Input: part model. Units: mm. Frame: model coordinates. Face numbers are marked on the shaded views. A direction names the side the tool comes from. Round coordinates to 2 decimals unless told otherwise and drop trailing zeros. Loops run counter-clockwise (first coordinate to the right, second up) from the corner with the lowest first, then second, coordinate; pieces in that order, holes last. Notation, with made-up numbers: M 18.25,0.25 L 48.25,0.25 A19 ccw 48.25,36.25 Z; hole C -27,24 d6. An arc over 180 degrees is marked long. Put each result on its own line as item: value. Start each with the question number.
1) Section C-C on x = 80. Output: boundary loops of the cut face in (y, z), plus the area to 3 significant figures.
2) Section A-A on y = 0. Output: boundary loops of the cut face in (x, z), plus the area to 3 significant figures.
3) Reachability of the marked faces 1 and 2 from +Z, -Z, +X, -X, +Y, -Y: full face, straight path, thin tool, end or side. Return the list, or none.
4) Line query: probe 1 along X at (y, z) = (7, 26.5); probe 2 along Y at (x, z) = (52.5, -0.5); probe 3 along X at (y, z) = (-1, 31). Output: solid intervals per line, ascending.
5) Draft query along X for the marked faces 3, 4, 5 and 6. Return one class per face: +X half, -X half, draft (parallel to the pull), parting line (faces both ways), or undercut.
6) Section B-B on z = 21.5. Output: boundary loops of the cut face in (x, y), plus the area to 3 significant figures.
7) Pin query (flat end, axial travel): pin 1 (14.5 mm diameter, centred on y = -3, z = 0.5, fed in from -X); pin 2 (1.5 mm diameter, centred on x = 19, z = -4, fed in from -Y); pin 3 (8 mm diameter, centred on x = 7.5, z = 22.5, fed in from +Y). Return the tip coordinate at first contact, or that it passes through.
from build123d import *

# Parameters (mm, degrees)
F1_DEPTH = 36.576
F2_R     = 6.1269141817
F2_R_2   = 5.4449422531
F3_DEPTH = 42.418
F4_DEPTH = 25.4
F5_DEPTH = 25.4
F6_R     = 11.6411765601
F7_DEPTH = 33.528


with BuildPart() as f1:
    # F0 (on Right) → F1 (new body)
    with BuildSketch(Plane.YZ):
        with BuildLine():
            ThreePointArc((-7.3964224414, -6.1888854819), (3.2922075385, -9.0648076628), (9.6441364797, 0))
            ThreePointArc((9.6441364797, 0), (3.2922075385, 9.0648076628), (-7.3964224414, 6.1888854819))
            ThreePointArc((-7.3964224414, 6.1888854819), (-4.251808406, 3.7785340877), (-3.0597214027, 0))
            ThreePointArc((-3.0597214027, 0), (-4.251808406, -3.7785340877), (-7.3964224414, -6.1888854819))
        make_face()
        with BuildLine():
            ThreePointArc((-3.0597214027, 0), (-4.251808406, 3.7785340877), (-7.3964224414, 6.1888854819))
            ThreePointArc((-7.3964224414, 6.1888854819), (-9.6441364797, 0), (-7.3964224414, -6.1888854819))
            ThreePointArc((-7.3964224414, -6.1888854819), (-4.251808406, -3.7785340877), (-3.0597214027, 0))
        make_face()
        with BuildLine():
            ThreePointArc((-7.3964224414, -6.1888854819), (-9.6441364797, 0), (-7.3964224414, 6.1888854819))
            ThreePointArc((-7.3964224414, 6.1888854819), (-16.2285515567, 0), (-7.3964224414, -6.1888854819))
        make_face()
    extrude(amount=F1_DEPTH)

    # F2 (on Top) → F3 (join)
    with BuildSketch(Plane.XY):
        with Locations((10.4273650795, 0)):
            Circle(F2_R)
        with Locations((10.4273650795, 0)):
            Circle(F2_R_2, mode=Mode.SUBTRACT)
    extrude(amount=F3_DEPTH)

    # F4 (add): a face of the model
    f4_faces = [f1.faces().sort_by_distance(p)[0] for p in [
        (36.576, -2.5293914457, 0),
    ]]
    extrude(f4_faces, amount=F4_DEPTH)

    # F5 (add): a face of the model
    f5_faces = [f1.faces().sort_by_distance(p)[0] for p in [
        (61.976, -2.5293914457, 0),
    ]]
    extrude(f5_faces, amount=F5_DEPTH)

    # F6 (on Top) → F7 (join)
    with BuildSketch(Plane.XY):
        with Locations((0, 6.7043649033)):
            Circle(F6_R)
    extrude(amount=F7_DEPTH)


solid = f1.part
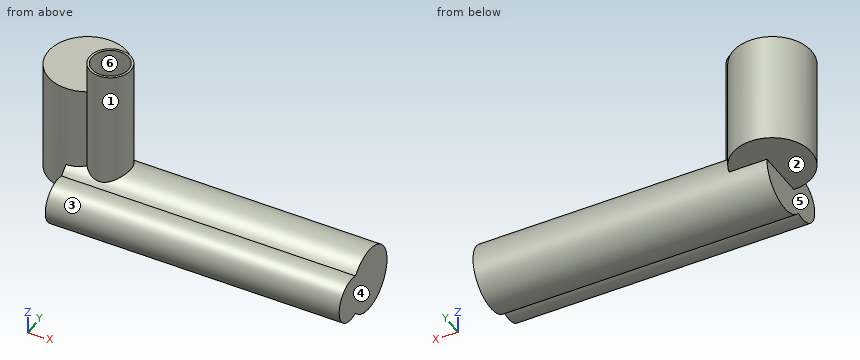
Geometry results:
1. outline: M -7.4,-6.19 A9.64 ccw long -7.4,6.19 A6.58 ccw long Z
1. area: 370 mm²
2. outline: M -9.52,0 L 0,0 L 0,-9.64 L 87.38,-9.64 L 87.38,9.64 L 16.55,9.64 L 16.55,42.42 L 15.87,42.42 L 15.87,9.64 L 9.52,9.64 L 9.52,33.53 L 4.98,33.53 L 4.98,42.42 L 4.3,42.42 L 4.3,33.53 L -9.52,33.53 Z
2. area: 2,260 mm²
3. face 1: +Z
3. face 2: -Z, -X, +Y
4. probe 1: x = -11.64 to 11.64
4. probe 2: y = -16.21 to 9.63
4. probe 3: x = -8.73 to 8.73, 15.78 to 16.47
5. face 3: draft
5. face 4: +X half
5. face 5: -X half
5. face 6: undercut
6. outline: M 5.45,-3.58 A6.13 ccw long 11.62,6.01 A11.64 ccw long Z; hole M 6.05,-3.24 A5.44 ccw long 11.56,5.33 A11.64 cw Z
6. area: 441 mm²
7. pin 1: stops at x = -11.38
7. pin 2: stops at y = -15.37
7. pin 3: stops at y = 17.81
